The listing builds one solid part. Answer for the finished solid, in the listing's coordinates (mm). Face numbers are marked on the shaded views. A direction names the side the tool comes from. Round coordinates to 2 decimals unless told otherwise and drop trailing zeros. Order: outer loops, then holes, each group sorted by start corner. A loop starts at its lowest first (then second) coordinate and runs counter-clockwise, first axis right, second up. Notation, with made-up numbers: (86.25, -12) -> (128.25, -12) arc R25 cw to (128.25, 17) -> close; hole circle Ø11 at (25.25, -11). An arc over 180 degrees is marked (long way). Answer in a Markdown table with one row per item. Add a question column.
```python
from build123d import *

# Parameters (mm, degrees)
SKETCH1_W           = 100
SKETCH1_H           = 100
BOSS_EXTRUDE1_DEPTH = 35


with BuildPart() as part:
    # Sketch1 → Boss-Extrude1 (new body)
    with BuildSketch(Plane.XY):
        Rectangle(SKETCH1_W, SKETCH1_H)
    extrude(amount=BOSS_EXTRUDE1_DEPTH)

    # Sketch2 → Revolve1 (revolve)
    with BuildSketch(Plane(origin=(0, 0, 0), x_dir=(1, 0, 0), z_dir=(0, 1, 0))):
        with BuildLine():
            Line((0, -35), (0, -72.5))
            Line((0, -72.5), (0, -85))
            ThreePointArc((0, -85), (11.469869254, -77.469114539), (9.119215052, -63.950735889))
            Line((9.119215052, -63.950735889), (40, -35))
            Line((40, -35), (0, -35))
        make_face()
    revolve(axis=Axis((0, 0, 35), (0, 0, 1)))


solid = part.part
```
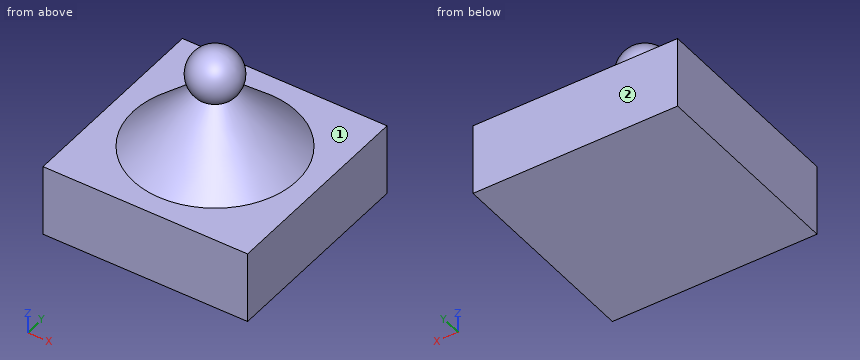
1. Straight lines are drawn through the part: line 1 along Z through (x, y) = (-44, 24); line 2 along X through (y, z) = (3, 74.5); line 3 along X through (y, z) = (-17.5, 40). For each, find the intervals that lie inside material, in ascending order.
2. For the marked faces 1 and 2, determine the directions among +Z, -Z, +X, -X, +Y, -Y from which every point of the face is accessible in a straight line to the end or side of a thin tool.
3. The part is cut by section D-D (z = 67). Give the vertices of the cut face in (x, y).
4. The part is cut by section A-A (y = 0). Give the vertices of the cut face in (x, z).
5. Each of these flat-tipped pins is pushed along its axis until it touches: pin 1 (1.5 mm diameter, centred on x = -9.5, y = 25.5, fed in from +Z); pin 2 (4 mm diameter, centred on x = -29, y = 29.5, fed in from -Z); pin 3 (8 mm diameter, centred on x = -15, z = 57.5, fed in from +Y); pin 4 (6 mm diameter, centred on x = -11.5, y = 9, fed in from +Z). Where does it stop, or does it pass through?
6. The part is cut by section C-C (z = 46). Give the vertices of the cut face in (x, y).
Report:
| question | item | result |
|---|---|---|
| 1 | line 1 | z = 0 to 35 |
| 1 | line 2 | x = -11.97 to 11.97 |
| 1 | line 3 | x = -29.93 to 29.93 |
| 2 | face 1 | +Z |
| 2 | face 2 | +Z, -Z, +X, -X, +Y |
| 3 | outline | circle Ø22.45 at (0, 0) |
| 4 | outline | (-50, 0) -> (50, 0) -> (50, 35) -> (40, 35) -> (9.12, 63.95) arc R12.5 ccw (long way) to (-9.12, 63.95) -> (-40, 35) -> (-50, 35) -> close |
| 5 | pin 1 | stops at z = 47.69 |
| 5 | pin 2 | stops at z = 0 |
| 5 | pin 3 | stops at y = 14.8 |
| 5 | pin 4 | stops at z = 77.15 |
| 6 | outline | circle Ø56.53 at (0, 0) |
